Part model, mm, in its own coordinate system. A direction names the side the tool comes from. Round coordinates to 2 decimals unless told otherwise and drop trailing zeros. Write each loop counter-clockwise with the first axis right and the second up, starting at its lowest first coordinate (ties: lowest second). Pieces come first, ordered by that corner, then holes. Notation, with made-up numbers: M 61.25,-31 L 77.25,-31 A29 cw 77.25,-7 Z; hole C 19,43.5 d8. An arc over 180 degrees is marked long. Answer as a JSON object with one key per item and string values. Group by question number.
1. Drop flat-ended pins along their axis: pin 1 (2.5 mm diameter, centred on y = 34.4, z = 5, fed in from -X); pin 2 (8 mm diameter, centred on y = 25, z = 47.5, fed in from +X); pin 3 (10 mm diameter, centred on x = 24.5, z = 42.5, fed in from +Y). Give the stop position or say it passes through.
2. Band-saw the part on C-C, the plane z = 9.75. Write the cut outline in (x, y).
3. Band-saw the part on A-A, the plane z = 34. Write the cut outline in (x, y), plus the area to 3 significant figures.
4. Which spindle directions (+Z, -Z, +X, -X, +Y, -Y) get a long thin tool onto all of the face, cutting with end or side? Do faces 5 (the face through (-10.49, -20.43, 22)), 6 (the face through (-5.419, -1, 34)). Say none if no direction does.
5. Band-saw the part on D-D, the plane y = -6.5. Write the cut outline in (x, z).
6. Band-saw the part on B-B, the plane z = 44.5. Write the cut outline in (x, y).
7. Two-plate mould, pull along X, no slides. Class faces 1 (the face through (59.581, -46, 34)), 2 (the face through (45.39, -45.64, 54.69)), 3 (the face through (-10.489, 33.825, 64.386)), 4 (the face through (-15.419, 0, 34)): +X half, -X half, draft (parallel to the pull), parting line (faces both ways), or undercut.
8. Drill centre lines: line 1 (Y direction, x = -10.5, z = 44.5); line 2 (Y direction, x = -8.75, z = 9.75); line 3 (Y direction, x = -8.5, z = 34). Where is each one in solid material? Low to high. Write a range as from..to.
from build123d import *

# Parameters (mm, degrees)
EXTRUDE_1_DEPTH     = 68
SKETCH_2_R          = 2.5
CUT_EXTRUDE_1_DEPTH = 76
FILLET_1_R          = 5
FILLET_3_R          = 5
SKETCH_7_R          = 1.5
CUT_EXTRUDE_5_DEPTH = 10
SKETCH_8_R          = 1.5
CUT_EXTRUDE_6_DEPTH = 10
SKETCH_9_R          = 1.5
CUT_EXTRUDE_7_DEPTH = 10
FILLET_4_R          = 2.5
SKETCH_14_R         = 2
SKETCH_14_R_2       = 1.5
SKETCH_14_R_3       = 4
CUT_EXTRUDE_9_DEPTH = 76


with BuildPart() as part:
    # 草图1 → 凸台-拉伸1 (new body)
    with BuildSketch(Plane.XY):
        Polygon((-15.418994413, 41.899441341), (-15.418994413, -48.100558659), (59.581005587, -48.100558659), (59.581005587, -43.100558659), (-5.418994413, -43.100558659), (-5.418994413, 41.899441341), align=None)
    extrude(amount=EXTRUDE_1_DEPTH)

    # 草图2 → 切除-拉伸1 (cut, through all)
    with BuildSketch(Plane.ZY.offset(15.418994413)):
        with Locations((34, 9.399441341)):
            Circle(SKETCH_2_R)
    extrude(amount=-CUT_EXTRUDE_1_DEPTH, mode=Mode.SUBTRACT)

    # 圆角1
    fillet_1_edges = [part.edges().sort_by_distance(p)[0] for p in [
        (-10.418994413, 41.899441341, 68),
        (-10.418994413, 41.899441341, 0),
    ]]
    fillet(fillet_1_edges, radius=FILLET_1_R)

    # 圆角3
    fillet_3_edges = [part.edges().sort_by_distance(p)[0] for p in [
        (-15.418994413, -48.100558659, 34),
    ]]
    fillet(fillet_3_edges, radius=FILLET_3_R)

    # 草图7 → 切除-拉伸5 (cut)
    with BuildSketch(Plane.ZY.offset(15.418994413)):
        with Locations((63, 34.399441341)):
            Circle(SKETCH_7_R)
        with Locations((5, 34.399441341)):
            Circle(SKETCH_7_R)
    extrude(amount=-CUT_EXTRUDE_5_DEPTH, mode=Mode.SUBTRACT)

    # 草图8 → 切除-拉伸6 (cut)
    with BuildSketch(Plane.XZ.offset(48.100558659)):
        with Locations((44.581005587, 14.571428571)):
            Circle(SKETCH_8_R)
        with Locations((44.581005587, 53.428571429)):
            Circle(SKETCH_8_R)
    extrude(amount=-CUT_EXTRUDE_6_DEPTH, mode=Mode.SUBTRACT)

    # 草图9 → 切除-拉伸7 (cut)
    with BuildSketch(Plane.ZY.offset(15.418994413)):
        with Locations((5, -38.100558659)):
            Circle(SKETCH_9_R)
        with Locations((63, -38.100558659)):
            Circle(SKETCH_9_R)
    extrude(amount=-CUT_EXTRUDE_7_DEPTH, mode=Mode.SUBTRACT)

    # 圆角4
    fillet_4_edges = [part.edges().sort_by_distance(p)[0] for p in [
        (59.581005587, -45.600558659, 68),
        (59.581005587, -45.600558659, 0),
    ]]
    fillet(fillet_4_edges, radius=FILLET_4_R)

    # 草图14 → 切除-拉伸9 (cut, through all)
    with BuildSketch(Plane.ZY.offset(15.418994413)):
        with Locations((58.25, -27.496370313)):
            Circle(SKETCH_14_R)
        with Locations((58.25, -17.496370313)):
            Circle(SKETCH_14_R)
        with Locations((9.75, -17.496370313)):
            Circle(SKETCH_14_R)
        with Locations((9.75, -27.496370313)):
            Circle(SKETCH_14_R)
        with Locations((23.5, -34.496370313)):
            Circle(SKETCH_14_R_2)
        with Locations((44.5, -27.496370313)):
            Circle(SKETCH_14_R_3)
        with Locations((23.5, -27.496370313)):
            Circle(SKETCH_14_R_3)
        with Locations((34, -16.996370313)):
            Circle(SKETCH_14_R_3)
        with Locations((44.5, -20.496370313)):
            Circle(SKETCH_14_R_2)
        with Locations((51.5, -27.496370313)):
            Circle(SKETCH_14_R_2)
        with Locations((44.5, -34.496370313)):
            Circle(SKETCH_14_R_2)
        with Locations((16.5, -27.496370313)):
            Circle(SKETCH_14_R_2)
        with Locations((23.5, -20.496370313)):
            Circle(SKETCH_14_R_2)
        with Locations((30.5, -27.496370313)):
            Circle(SKETCH_14_R_2)
        with Locations((27, -16.996370313)):
            Circle(SKETCH_14_R_2)
        with Locations((34, -9.996370313)):
            Circle(SKETCH_14_R_2)
        with Locations((41, -16.996370313)):
            Circle(SKETCH_14_R_2)
        with Locations((34, -23.996370313)):
            Circle(SKETCH_14_R_2)
        with Locations((37.5, -27.496370313)):
            Circle(SKETCH_14_R_2)
    extrude(amount=-CUT_EXTRUDE_9_DEPTH, mode=Mode.SUBTRACT)


solid = part.part
Worked answers:
{
 "1": {"pin 1": "passes through", "pin 2": "stops at x = -5.42", "pin 3": "stops at y = -43.1"},
 "2": {"outline": "M -15.42,-43.1 A5 ccw -10.42,-48.1 L 59.58,-48.1 L 59.58,-43.1 L -5.42,-43.1 L -5.42,-29.5 L -15.42,-29.5 Z; M -15.42,-25.5 L -5.42,-25.5 L -5.42,-19.5 L -15.42,-19.5 Z; M -15.42,-15.5 L -5.42,-15.5 L -5.42,41.9 L -15.42,41.9 Z"},
 "3": {"outline": "M -15.42,-43.1 A5 ccw -10.42,-48.1 L 59.58,-48.1 L 59.58,-43.1 L -5.42,-43.1 L -5.42,-25.5 L -15.42,-25.5 Z; M -15.42,-22.5 L -5.42,-22.5 L -5.42,-21 L -15.42,-21 Z; M -15.42,-13 L -5.42,-13 L -5.42,-11.5 L -15.42,-11.5 Z; M -15.42,-8.5 L -5.42,-8.5 L -5.42,6.9 L -15.42,6.9 Z; M -15.42,11.9 L -5.42,11.9 L -5.42,41.9 L -15.42,41.9 Z", "area": "1,030 mm^2"},
 "4": {"face 5": "+X, -X", "face 6": "+Z, -Z, +X, +Y"},
 "5": {"outline": "M -15.42,0 L -5.42,0 L -5.42,68 L -15.42,68 Z"},
 "6": {"outline": "M -15.42,-43.1 A5 ccw -10.42,-48.1 L 59.58,-48.1 L 59.58,-43.1 L -5.42,-43.1 L -5.42,-36 L -15.42,-36 Z; M -15.42,-33 L -5.42,-33 L -5.42,-31.5 L -15.42,-31.5 Z; M -15.42,-23.5 L -5.42,-23.5 L -5.42,-22 L -15.42,-22 Z; M -15.42,-19 L -5.42,-19 L -5.42,41.9 L -15.42,41.9 Z"},
 "7": {"face 1": "+X half", "face 2": "undercut", "face 3": "draft", "face 4": "-X half"},
 "8": {"line 1": "y = -48.1..-36, -33..-31.5, -23.5..-22, -19..41.9", "line 2": "y = -48.1..-29.5, -25.5..-19.5, -15.5..41.9", "line 3": "y = -48.1..-25.5, -22.5..-21, -13..-11.5, -8.5..6.9, 11.9..41.9"}
}
